from build123d import *

# Parameters (mm, degrees)
BOSS_EXTRUDE1_DEPTH = 20
SKETCH2_R           = 2
CUT_EXTRUDE1_DEPTH  = 59.51709152
FILLET1_R           = 6
FILLET2_R           = 6
FILLET3_R           = 2
FILLET4_R           = 2


with BuildPart() as part:
    # Sketch1 → Boss-Extrude1 (new body)
    with BuildSketch(Plane(origin=(0, 0, 0), x_dir=(1, 0, 0), z_dir=(0, 1, 0))):
        Polygon((-35.5, 0), (-21, 0), (-21, 36), (-15, 42), (15, 42), (21, 36), (21, 0), (35.5, 0), (35.5, 2.5), (23.5, 2.5), (23.5, 37.035533906), (16.035533906, 44.5), (-16.035533906, 44.5), (-23.5, 37.035533906), (-23.5, 2.5), (-35.5, 2.5), align=None)
    extrude(amount=BOSS_EXTRUDE1_DEPTH)

    # Sketch2 → Cut-Extrude1 (cut, through all)
    with BuildSketch(Plane(origin=(0, 0, -2.5), x_dir=(-1, 0, 0), z_dir=(0, 0, -1))):
        with Locations((29.5, 14.5)):
            Circle(SKETCH2_R)
        with Locations((29.5, 5.5)):
            Circle(SKETCH2_R)
    cut_extrude1 = extrude(amount=-CUT_EXTRUDE1_DEPTH, mode=Mode.SUBTRACT)

    # Mirror1: Cut-Extrude1 across plane
    add(cut_extrude1.mirror(Plane(origin=(0, 0, 0), x_dir=(0, 0, 1), z_dir=(1, 0, 0))), mode=Mode.SUBTRACT)

    # Fillet1
    fillet1_edges = [part.edges().sort_by_distance(p)[0] for p in [
        (-16.035533906, 10, -44.5),
        (16.035533906, 10, -44.5),
        (23.5, 10, -37.035533906),
        (-23.5, 10, -37.035533906),
    ]]
    fillet(fillet1_edges, radius=FILLET1_R)

    # Fillet2
    fillet2_edges = [part.edges().sort_by_distance(p)[0] for p in [
        (21, 10, -36),
        (15, 10, -42),
        (-15, 10, -42),
        (-21, 10, -36),
    ]]
    fillet(fillet2_edges, radius=FILLET2_R)

    # Fillet3
    fillet3_edges = [part.edges().sort_by_distance(p)[0] for p in [
        (23.5, 10, -2.5),
        (-23.5, 10, -2.5),
    ]]
    fillet(fillet3_edges, radius=FILLET3_R)

    # Fillet4
    fillet4_edges = [part.edges().sort_by_distance(p)[0] for p in [
        (-35.5, 20, -1.25),
        (35.5, 0, -1.25),
        (-35.5, 0, -1.25),
        (35.5, 20, -1.25),
    ]]
    fillet(fillet4_edges, radius=FILLET4_R)


solid = part.part
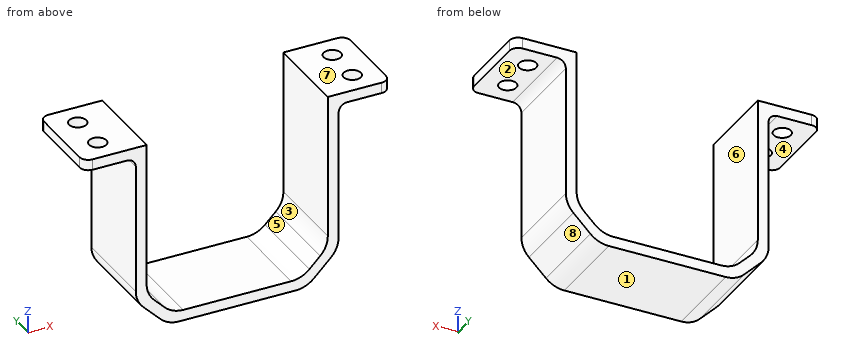
Could you check a few things on this model? Use its own coordinates, in mm. Face numbers are marked on the shaded views. A direction names the side the tool comes from. Coordinates: 2 decimals unless noted, no trailing zeros. Loops run counter-clockwise (first coordinate to the right, second up) from the corner with the lowest first, then second, coordinate; pieces in that order, holes last. Notation, with made-up numbers: (-32, -22) -> (20, -22) arc R19 ccw to (20, 14) -> close; hole circle Ø4 at (58.5, 14.25). An arc over 180 degrees is marked (long way). Answer in a Markdown table with one row per item.
(1) Imagine slicing it at B-B (z = -15). List the corners of the cut face in (x, y) for me.
Results found:
| item | result |
|---|---|
| outline | (-23.5, 0) -> (-21, 0) -> (-21, 20) -> (-23.5, 20) -> close; (21, 0) -> (23.5, 0) -> (23.5, 20) -> (21, 20) -> close |
(2) Imagine slicing it at D-D (x = 9). List the corners of the cut face in (y, z) for me.
Results found:
| item | result |
|---|---|
| outline | (0, -44.5) -> (20, -44.5) -> (20, -42) -> (0, -42) -> close |
(3) Imagine slicing it at A-A (x = 29.5). List the corners of the cut face in (y, z) for me, plus the area to 3 significant figures.
Results found:
| item | result |
|---|---|
| outline | (0, -2.5) -> (3.5, -2.5) -> (3.5, 0) -> (0, 0) -> close; (7.5, -2.5) -> (12.5, -2.5) -> (12.5, 0) -> (7.5, 0) -> close; (16.5, -2.5) -> (20, -2.5) -> (20, 0) -> (16.5, 0) -> close |
| area | 30.0 mm^2 |
(4) If I drill on probe 1 along Y at (x, z) = (-29.5, -1.1); probe 2 along X at (y, z) = (7.5, -22.5); probe 3 along Y at (x, z) = (-29, -1), over which ranges is the centre line in solid material (lowest first)?
Results found:
| item | result |
|---|---|
| probe 1 | y = 0 to 3.5, 7.5 to 12.5, 16.5 to 20 |
| probe 2 | x = -23.5 to -21, 21 to 23.5 |
| probe 3 | y = 0 to 3.56, 7.44 to 12.56, 16.44 to 20 |
(5) Thinking about a two-plate mould opening in X: for the marked faces 5, 6, 7 and 8, which applies, released by +X, released by -X, zero draft, split by the parting line, or undercut?
Results found:
| item | result |
|---|---|
| face 5 | undercut |
| face 6 | undercut |
| face 7 | zero draft |
| face 8 | released by +X |
(6) Will these pins go through, and if not, where does the flat tip stop? pin 1 Ø6 at (y, z) = (9.5, -21.5) entering from -X; pin 2 Ø8 at (x, y) = (-32.5, 13) entering from -Z; pin 3 Ø2 at (x, y) = (-2.5, 13) entering from +Z.
Results found:
| item | result |
|---|---|
| pin 1 | stops at x = -23.5 |
| pin 2 | stops at z = -2.5 |
| pin 3 | stops at z = -42 |
(7) For the marked faces 1, 2, 3 and 4, which set-ups out of +Z, -Z, +X, -X, +Y, -Y let a thin tool reach every point of the face, with its end or its side?
Results found:
| item | result |
|---|---|
| face 1 | -Z, +X, -X, +Y, -Y |
| face 2 | -Z, +X, +Y, -Y |
| face 3 | +Z, +Y, -Y |
| face 4 | -Z, -X, +Y, -Y |
(8) Imagine slicing it at C-C (y = 14.5). Give the number of separate pieces and of enclosed holes in the cut face, plus the area to 3 significant figures.
Results found:
| item | result |
|---|---|
| separate pieces | 3 |
| enclosed holes | 0 |
| area | 349 mm^2 |
